Check sheet for the drawn part. Datum: minimum x, y, z corner. Units: mm. A direction names the side the tool comes from. Round coordinates to 2 decimals unless told otherwise and drop trailing zeros. Order: outer loops, then holes, each group sorted by start corner. A loop starts at its lowest first (then second) coordinate and runs counter-clockwise, first axis right, second up. Notation, with made-up numbers: (-1.75, 89.25) -> (9.25, 89.25) arc R23 ccw to (9.25, 110.25) -> close; hole circle Ø7 at (6.5, 49). An arc over 180 degrees is marked (long way). Use CSV: the item, a comma, the result in double quotes.
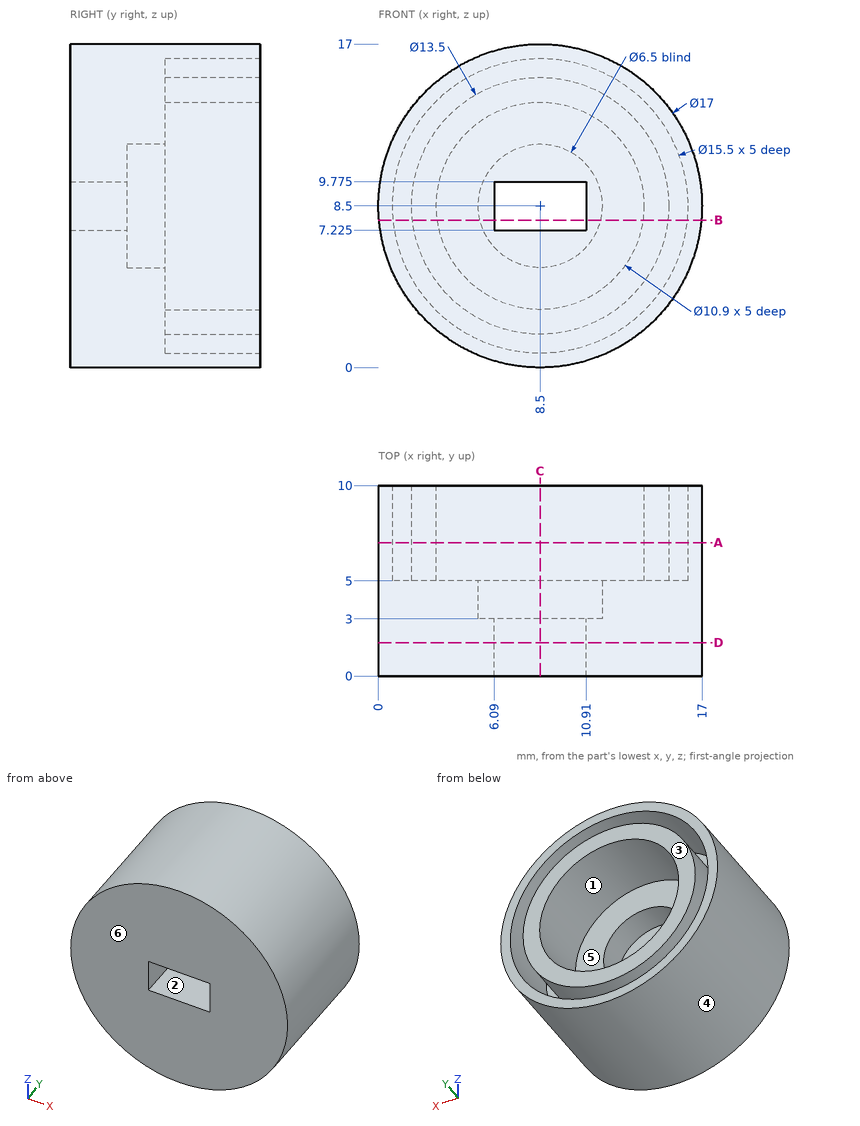
Q1. Sectioned sample at D-D, the plane y = 1.75. Enter the section's corners in (x, z) (3 decimals).
Result sheet:
outline,"circle Ø17 at (8.5, 8.5); hole (6.09, 7.225) -> (10.91, 7.225) -> (10.91, 9.775) -> (6.09, 9.775) -> close"
Q2. Go/stop test with flat-tipped pins: pin 1 (1 mm diameter, centred on y = 2, z = 9.5, fed in from -X); pin 2 (3 mm diameter, centred on x = 3.5, y = 8, fed in from -Z); pin 3 (2 mm diameter, centred on y = 3, z = 6.5, fed in from +X); pin 4 (0.8 mm diameter, centred on y = 1, z = 8, fed in from +X). Record where each tip stops, or that it passes through.
Result sheet:
pin 1,"stops at x = 0.01"
pin 2,"stops at z = 0.75"
pin 3,"stops at x = 16.94"
pin 4,"stops at x = 17"
Q3. Sectioned sample at B-B, the plane z = 7.75. Enter the section's corners in (x, y), then the cut area to 3 significant figures.
Result sheet:
outline,"(0.03, 0) -> (6.09, 0) -> (6.09, 3) -> (5.34, 3) -> (5.34, 5) -> (3.1, 5) -> (3.1, 10) -> (1.79, 10) -> (1.79, 5) -> (0.79, 5) -> (0.79, 10) -> (0.03, 10) -> close; (10.91, 0) -> (16.97, 0) -> (16.97, 10) -> (16.21, 10) -> (16.21, 5) -> (15.21, 5) -> (15.21, 10) -> (13.9, 10) -> (13.9, 5) -> (11.66, 5) -> (11.66, 3) -> (10.91, 3) -> close"
area,"78.2 mm^2"
Q4. Scan lines: L1, parallel to X at y = 6.2, z = 8.5; L2, parallel to Z at x = 8.5, y = 4.15; L3, parallel to Z at x = 8.75, y = 5.75. Record each from-to range of solid material in increasing order.
Result sheet:
L1,"x = 0 to 0.75, 1.75 to 3.05, 13.95 to 15.25, 16.25 to 17"
L2,"z = 0 to 5.25, 11.75 to 17"
L3,"z = 0 to 0.75, 1.75 to 3.06, 13.94 to 15.25, 16.25 to 17"
Q5. Access from +Z, -Z, +X, -X, +Y, -Y to the whole of each face (thin tool, end or side, straight path). Record for the marked faces 1, 2 and 3.
Result sheet:
face 1,"+Y"
face 2,"+Y, -Y"
face 3,"+Z, -Z, +X, -X, +Y"
Q6. Sectioned sample at C-C, the plane x = 8.5. Enter the section's corners in (y, z) (3 decimals).
Result sheet:
outline,"(0, 0) -> (10, 0) -> (10, 0.75) -> (5, 0.75) -> (5, 1.75) -> (10, 1.75) -> (10, 3.05) -> (5, 3.05) -> (5, 5.25) -> (3, 5.25) -> (3, 7.225) -> (0, 7.225) -> close; (0, 9.775) -> (3, 9.775) -> (3, 11.75) -> (5, 11.75) -> (5, 13.95) -> (10, 13.95) -> (10, 15.25) -> (5, 15.25) -> (5, 16.25) -> (10, 16.25) -> (10, 17) -> (0, 17) -> close"
Q7. Mould release check, pull along X, two halves, no side actions. Record for the marked faces 4, 5 and 6: pulls with the +X half, pulls with the -X half, needs draft (parallel to the pull), parting line crosses it, or undercut.
Result sheet:
face 4,"parting line crosses it"
face 5,"undercut"
face 6,"needs draft"
Q8. Sectioned sample at A-A, the plane y = 7. Enter the section's corners in (x, z), then the cut area to 3 significant figures.
Result sheet:
outline,"circle Ø17 at (8.5, 8.5); circle Ø13.5 at (8.5, 8.5); hole circle Ø15.5 at (8.5, 8.5); hole circle Ø10.9 at (8.5, 8.5)"
area,"88.1 mm^2"
